For this review, take the finished solid that the model builds, in its own axes (mm). A direction names the side the tool comes from. Round coordinates to 2 decimals unless told otherwise and drop trailing zeros. Order: outer loops, then holes, each group sorted by start corner. A loop starts at its lowest first (then second) coordinate and runs counter-clockwise, first axis right, second up. Notation, with made-up numbers: (-13, -29) - (25, -29) arc R14 ccw to (25, -9) - close; hole circle Ø7 at (73, 73.5). An arc over 180 degrees is marked (long way). One line per question, with ' | ' between items.
```python
from build123d import *

# Parameters (mm, degrees)
BOSS_EXTRUDE1_DEPTH = 10
SKETCH1_3_OUTSIDE_W = 885.69
SKETCH1_3_OUTSIDE_H = 260.69
SKETCH1_3_OUTSIDE_R = 30
CUT_EXTRUDE1_DEPTH  = 3
SKETCH1_5_R         = 30
CUT_EXTRUDE3_DEPTH  = 10
SKETCH1_6_R         = 30
SKETCH1_6_R_2       = 20
BOSS_EXTRUDE2_DEPTH = 3
SKETCH1_7_R         = 30
CUT_EXTRUDE4_DEPTH  = 10
SKETCH1_8_R         = 30
SKETCH1_8_R_2       = 20
BOSS_EXTRUDE3_DEPTH = 3


with BuildPart() as part:
    # Sketch1 → Boss-Extrude1 (new, symmetric)
    with BuildSketch(Plane(origin=(0, 0, 0), x_dir=(1, 0, 0), z_dir=(0, 1, 0))):
        with BuildLine():
            Line((0, 55), (625, 55))
            ThreePointArc((625, 55), (680, 0), (625, -55))
            Line((625, -55), (0, -55))
            ThreePointArc((0, -55), (-55, 0), (0, 55))
        make_face()
    extrude(amount=BOSS_EXTRUDE1_DEPTH, both=True)

    # Sketch1<3> outside → Cut-Extrude1 (cut, symmetric)
    # profile 1 of 3: a face of its own
    with BuildSketch(Plane(origin=(0, 0, 0), x_dir=(1, 0, 0), z_dir=(0, 1, 0))):
        with Locations((312.5, 0)):
            Rectangle(SKETCH1_3_OUTSIDE_W, SKETCH1_3_OUTSIDE_H)
        with BuildLine():
            Line((0, 50), (625, 50))
            ThreePointArc((625, 50), (675, 0), (625, -50))
            Line((625, -50), (0, -50))
            ThreePointArc((0, -50), (-50, 0), (0, 50))
        make_face(mode=Mode.SUBTRACT)
    # profile 2 of 3: a face of its own
    with BuildSketch(Plane(origin=(0, 0, 0), x_dir=(1, 0, 0), z_dir=(0, 1, 0))):
        with Locations(Location((0, 0, 0), (0, 0, 270))):
            Circle(SKETCH1_3_OUTSIDE_R)
    # profile 3 of 3: a face of its own
    with BuildSketch(Plane(origin=(0, 0, 0), x_dir=(1, 0, 0), z_dir=(0, 1, 0))):
        with Locations(Location((625, 0, 0), (0, 0, 270))):
            Circle(SKETCH1_3_OUTSIDE_R)
    extrude(amount=CUT_EXTRUDE1_DEPTH, both=True, mode=Mode.SUBTRACT)

    # Sketch1<5> → Cut-Extrude3 (cut, symmetric)
    with BuildSketch(Plane(origin=(0, 0, 0), x_dir=(1, 0, 0), z_dir=(0, 1, 0))):
        with Locations(Location((625, 0, 0), (0, 0, 270))):
            Circle(SKETCH1_5_R)
    extrude(amount=CUT_EXTRUDE3_DEPTH, both=True, mode=Mode.SUBTRACT)

    # Sketch1<6> → Boss-Extrude2 (add, symmetric)
    with BuildSketch(Plane(origin=(0, 0, 0), x_dir=(1, 0, 0), z_dir=(0, 1, 0))):
        with Locations(Location((625, 0, 0), (0, 0, 270))):
            Circle(SKETCH1_6_R)
        with Locations(Location((625, 0, 0), (0, 0, 270))):
            Circle(SKETCH1_6_R_2, mode=Mode.SUBTRACT)
    extrude(amount=BOSS_EXTRUDE2_DEPTH, both=True)

    # Sketch1<7> → Cut-Extrude4 (cut, symmetric)
    with BuildSketch(Plane(origin=(0, 0, 0), x_dir=(1, 0, 0), z_dir=(0, 1, 0))):
        with Locations(Location((0, 0, 0), (0, 0, 270))):
            Circle(SKETCH1_7_R)
    extrude(amount=CUT_EXTRUDE4_DEPTH, both=True, mode=Mode.SUBTRACT)

    # Sketch1<8> → Boss-Extrude3 (add, symmetric)
    with BuildSketch(Plane(origin=(0, 0, 0), x_dir=(1, 0, 0), z_dir=(0, 1, 0))):
        with Locations(Location((0, 0, 0), (0, 0, 270))):
            Circle(SKETCH1_8_R)
        with Locations(Location((0, 0, 0), (0, 0, 270))):
            Circle(SKETCH1_8_R_2, mode=Mode.SUBTRACT)
    extrude(amount=BOSS_EXTRUDE3_DEPTH, both=True)


solid = part.part
```
(1) For probe 1 along X at (y, z) = (-6.75, 0); probe 2 along X at (y, z) = (-1.7, 0); probe 3 along Z at (x, y) = (293, 2.5), list the stretches that pass through material, from the lowest coordinate up. Write a range as [from, to].
Output values:
probe 1: [-55, -30], [30, 595], [655, 680] | probe 2: [-50, -20], [20, 605], [645, 675] | probe 3: [-50, 50]
(2) For faces 1 (the cylindrical face through (1.32, 6.55, -29.97)), 2 (the cylindrical face through (679.987, -6.451, -1.209)), 3 (the cylindrical face through (654.745, -6.451, -3.905)), list the 3-axis set-ups (+Z, -Z, +X, -X, +Y, -Y) from which the entire face can be reached by the end or side of a thin tool; tool diameter is ignored.
Output values:
face 1: +Y | face 2: +X, +Y, -Y | face 3: -Y
(3) We need section C-C on z = -4. Give the number of separate pieces and of enclosed holes in the cut face, plus the area to 3 significant figures.
Output values:
separate pieces: 3 | enclosed holes: 0 | area: 12,500 mm^2
(4) We need section B-B on z = 37.5. State the section outline as (x, y) points, plus the area to 3 significant figures.
Output values:
outline: (-40.23, -10) - (665.23, -10) - (665.23, -3) - (658.07, -3) - (658.07, 3) - (665.23, 3) - (665.23, 10) - (-40.23, 10) - (-40.23, 3) - (-33.07, 3) - (-33.07, -3) - (-40.23, -3) - close | area: 14,000 mm^2
(5) We need section A-A on x = 143. State the section outline as (y, z) points, plus the area to 3 significant figures.
Output values:
outline: (-10, -55) - (-3, -55) - (-3, -50) - (3, -50) - (3, -55) - (10, -55) - (10, 55) - (3, 55) - (3, 50) - (-3, 50) - (-3, 55) - (-10, 55) - close | area: 2,140 mm^2
(6) Mouldability with a two-part tool opening along Y and no side actions: class faces 4 (the cylindrical face through (674.988, -0.042, -1.099)), 5 (the cylindrical face through (-19.524, -0.042, -4.336)), 6 (the flat face through (-20, -3, 6)) as released by +Y, released by -Y, zero draft, split by the parting line, or undercut.
Output values:
face 4: undercut | face 5: zero draft | face 6: released by -Y
(7) Insertion check: pin 1 (1.8 mm diameter, centred on x = 315, y = -1, fed in from +Z); pin 2 (1.5 mm diameter, centred on y = -7, z = 10, fed in from +X); pin 3 (1.8 mm diameter, centred on x = 168, y = 1, fed in from -Z). Each pin has a flat end and moves straight along its axis. Give the tip position at first contact, or say it passes through.
Output values:
pin 1: z = 50 | pin 2: x = 679.22 | pin 3: z = -50
